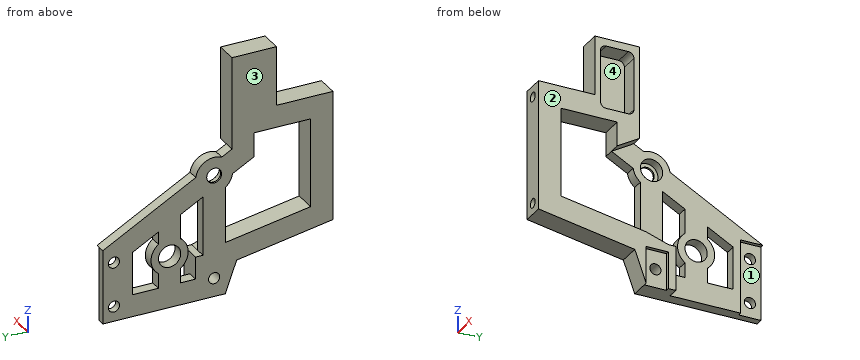
```python
from build123d import *

# Parameters (mm, degrees)
SKETCH1_R                   = 1.5
SKETCH1_R_2                 = 3
SKETCH1_R_3                 = 2
BOSS_EXTRUDE1_DEPTH         = 6
TAP_DRILL_FOR_M3_TAP1_D     = 2.5
TAP_DRILL_FOR_M3_TAP1_DEPTH = 9
TAP_DRILL_FOR_M3_TAP1_TIP   = 0.751075774
CUT_EXTRUDE4_DEPTH          = 3
SKETCH14_W                  = 20
SKETCH14_H                  = 6
CUT_EXTRUDE5_DEPTH          = 1
SKETCH15_W                  = 10
SKETCH15_H                  = 6
CUT_EXTRUDE6_DEPTH          = 1
SKETCH16_R                  = 3
CUT_EXTRUDE7_DEPTH          = 2.5
SKETCH17_W                  = 17
SKETCH17_H                  = 9
CUT_EXTRUDE8_DEPTH          = 5
FILLET1_R                   = 1.5


with BuildPart() as part:
    # Sketch1 → Boss-Extrude1 (new body)
    with BuildSketch(Plane(origin=(0, 0, 0), x_dir=(0, 0, -1), z_dir=(1, 0, 0))):
        with BuildLine():
            Line((51, 0), (55.572632785, 25.93268918))
            Line((55.572632785, 25.93268918), (64, 29))
            Line((64, 29), (64, 62))
            Line((64, 62), (44, 62))
            Line((44, 62), (30.288877114, 36.949172076))
            ThreePointArc((30.288877114, 36.949172076), (26.613988607, 34.400604937), (26.447909215, 29.931553848))
            Line((26.447909215, 29.931553848), (24.952842042, 27.2))
            Line((24.952842042, 27.2), (0, 27.2))
            Line((0, 27.2), (0, 15.2))
            Line((0, 15.2), (16, 15.2))
            Line((16, 15.2), (16, 0))
            Line((16, 0), (51, 0))
        make_face()
        with Locations((59, 32)):
            Circle(SKETCH1_R, mode=Mode.SUBTRACT)
        with Locations((50, 44)):
            Circle(SKETCH1_R_2, mode=Mode.SUBTRACT)
        with Locations((60, 59)):
            Circle(SKETCH1_R, mode=Mode.SUBTRACT)
        with Locations((48, 59)):
            Circle(SKETCH1_R, mode=Mode.SUBTRACT)
        with Locations((31, 32)):
            Circle(SKETCH1_R_3, mode=Mode.SUBTRACT)
        with BuildLine():
            Line((39.345952884, 41), (36.061960132, 35))
            Line((36.061960132, 35), (52, 35))
            Line((52, 35), (52, 37))
            Line((52, 37), (58, 37))
            Line((58, 37), (58, 41))
            Line((58, 41), (54, 41))
            ThreePointArc((54, 41), (50, 39), (46, 41))
            Line((46, 41), (39.345952884, 41))
        make_face(mode=Mode.SUBTRACT)
        with BuildLine():
            Line((46.461270512, 54), (42.629945635, 47))
            Line((42.629945635, 47), (46, 47))
            ThreePointArc((46, 47), (50, 49), (54, 47))
            Line((54, 47), (58, 47))
            Line((58, 47), (58, 54))
            Line((58, 54), (46.461270512, 54))
        make_face(mode=Mode.SUBTRACT)
        with BuildLine():
            Line((35, 29), (50.020922769, 29))
            Line((50.020922769, 29), (45.965402213, 6))
            Line((45.965402213, 6), (22, 6))
            Line((22, 6), (22, 21.2))
            Line((22, 21.2), (28.508776804, 21.2))
            Line((28.508776804, 21.2), (31.711122886, 27.050827924))
            ThreePointArc((31.711122886, 27.050827924), (33.549213145, 27.698661564), (35, 29))
        make_face(mode=Mode.SUBTRACT)
    extrude(amount=BOSS_EXTRUDE1_DEPTH)

    # Tap Drill for M3 Tap1
    with Locations(Plane(origin=(0, 0, 0), x_dir=(-1, 0, 0), z_dir=(0, -1, 0))):
        with Locations((-3, 48), (-3, 19)):
            Hole(TAP_DRILL_FOR_M3_TAP1_D / 2, depth=TAP_DRILL_FOR_M3_TAP1_DEPTH)
            with Locations((0, 0, -(TAP_DRILL_FOR_M3_TAP1_DEPTH + TAP_DRILL_FOR_M3_TAP1_TIP / 2))):  # 118° drill point
                Cone(0, TAP_DRILL_FOR_M3_TAP1_D / 2, TAP_DRILL_FOR_M3_TAP1_TIP, mode=Mode.SUBTRACT)

    # Sketch13 → Cut-Extrude4 (cut)
    with BuildSketch(Plane(origin=(6, 0, 0), x_dir=(0, 0, -1), z_dir=(1, 0, 0))):
        Polygon((52, 37), (64, 37), (64, 62), (44, 62), (30.288877114, 36.949172076), (28.008901276, 36.949172076), (23.767530455, 29.2), (28.508776804, 21.2), (50.020922769, 29), (52, 35), align=None)
    extrude(amount=-CUT_EXTRUDE4_DEPTH, mode=Mode.SUBTRACT)

    # Sketch14 → Cut-Extrude5 (cut)
    with BuildSketch(Plane(origin=(3, 0, 0), x_dir=(0, 0, -1), z_dir=(1, 0, 0))):
        with Locations((54, 59)):
            Rectangle(SKETCH14_W, SKETCH14_H)
    extrude(amount=-CUT_EXTRUDE5_DEPTH, mode=Mode.SUBTRACT)

    # Sketch15 → Cut-Extrude6 (cut)
    with BuildSketch(Plane(origin=(6, 0, 0), x_dir=(0, 0, -1), z_dir=(1, 0, 0))):
        with Locations((59, 32)):
            Rectangle(SKETCH15_W, SKETCH15_H)
    extrude(amount=-CUT_EXTRUDE6_DEPTH, mode=Mode.SUBTRACT)

    # Sketch16 → Cut-Extrude7 (cut)
    with BuildSketch(Plane(origin=(3, 0, 0), x_dir=(0, 0, -1), z_dir=(1, 0, 0))):
        with Locations((31, 32)):
            Circle(SKETCH16_R)
    extrude(amount=-CUT_EXTRUDE7_DEPTH, mode=Mode.SUBTRACT)

    # Sketch17 → Cut-Extrude8 (cut)
    with BuildSketch(Plane(origin=(6, 0, 0), x_dir=(0, 0, -1), z_dir=(1, 0, 0))):
        with Locations((10.5, 21.2)):
            Rectangle(SKETCH17_W, SKETCH17_H)
    extrude(amount=-CUT_EXTRUDE8_DEPTH, mode=Mode.SUBTRACT)

    # Fillet1
    fillet1_edges = [part.edges().sort_by_distance(p)[0] for p in [
        (3.5, 16.7, -2),
        (3.5, 25.7, -2),
        (3.5, 25.7, -19),
        (3.5, 16.7, -19),
    ]]
    fillet(fillet1_edges, radius=FILLET1_R)


solid = part.part
```
Check sheet for the modelled part. Datum: model origin and axes. Units: mm. Face numbers are marked on the shaded views. A direction names the side the tool comes from. Give positions to 0.01 mm unless a question says otherwise; leave off trailing zeros. Write each loop counter-clockwise with the first axis right and the second up, starting at its lowest first coordinate (ties: lowest second). Pieces come first, ordered by that corner, then holes.
Item 1: Gauge pin test, flat ends, axial feed: pin 1 (11.5 mm diameter, centred on y = 33.5, z = -48.5, fed in from +X); pin 2 (1 mm diameter, centred on x = 0.5, z = -14, fed in from +Y); pin 3 (1.5 mm diameter, centred on x = 4.5, z = -10, fed in from -Y). Record the tip position at first contact, or that the pin passes through.
Item 2: Cross-section at C-C (y = 44). Enter the section's corners in (x, z), and give its area (3 significant figures).
Item 3: Cross-section at A-A (y = 13). Enter the section's corners in (x, z).
Item 4: Cross-section at B-B (z = -15). Enter the section's corners in (x, y).
Item 5: Access from +Z, -Z, +X, -X, +Y, -Y to the whole of each face (thin tool, end or side, straight path). Record for the marked faces 1 and 2.
Item 6: Draft check along Z on the marked faces 3 and 4. Enter one of: released by +Z, released by -Z, zero draft, split by the parting line, or undercut.
Item 7: Scan lines: L1, parallel to Z at x = 0.4, y = 32; L2, parallel to Y at x = 1, z = -59; L3, parallel to Y at x = 2.2, z = -12. Record each from-to range of solid material in increasing order.
Report:
1. pin 1: stops at x = 6
1. pin 2: stops at y = 27.2
1. pin 3: stops at y = 15.2
2. outline: (0, -64) - (3, -64) - (3, -53) - (0, -53) - close; (0, -47) - (3, -47) - (3, -34.15) - (0, -34.15) - close
2. area: 71.6 mm2
3. outline: (0, -53.29) - (6, -53.29) - (6, -47.2) - (0, -47.2) - close; (0, -22) - (6, -22) - (6, -16) - (0, -16) - close
4. outline: (0, 15.2) - (6, 15.2) - (6, 16.7) - (1, 16.7) - (1, 25.7) - (6, 25.7) - (6, 27.2) - (0, 27.2) - close
5. face 1: -Z, +X, +Y
5. face 2: +Z, -Z, +X, +Y, -Y
6. face 3: zero draft
6. face 4: undercut
7. L1: z = -64 to -60.5, -57.5 to -33, -29 to -26
7. L2: y = 27.18 to 30.5, 33.5 to 57.88, 60.12 to 62
7. L3: y = 15.2 to 16.7, 25.7 to 27.2
